For this review, use the dimensioned drawing (mm, ordinates from the lowest corner) and the shaded views. A direction names the side the tool comes from. Coordinates: 2 decimals unless noted, no trailing zeros. Order: outer loops, then holes, each group sorted by start corner. A loop starts at its lowest first (then second) coordinate and runs counter-clockwise, first axis right, second up. Notation, with made-up numbers: M 70.5,-3 L 121.5,-3 A28 ccw 121.5,15 Z; hole C 54.25,72.5 d1. An arc over 180 degrees is marked long. Use CSV: the item, a comma, the result in double quotes.
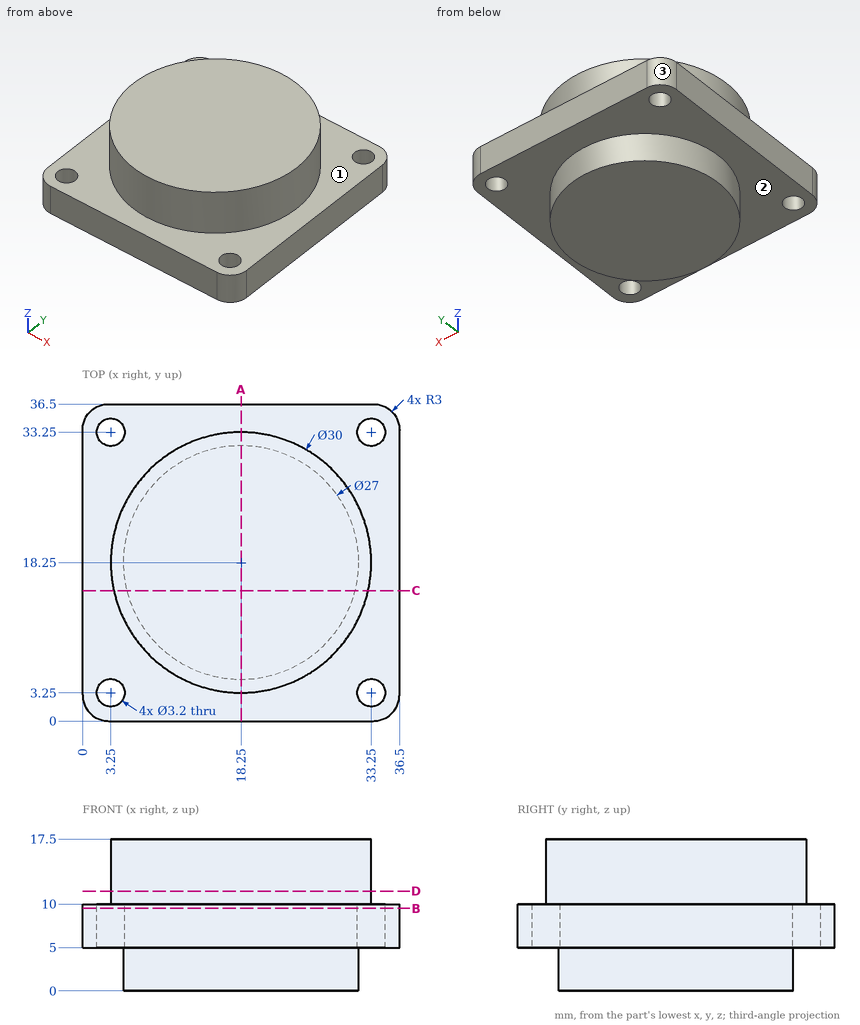
Item 1: Add section B-B on z = 9.5. State the section outline as (x, y) points.
Solutions:
outline,"M 0,3 A3 ccw 3,0 L 33.5,0 A3 ccw 36.5,3 L 36.5,33.5 A3 ccw 33.5,36.5 L 3,36.5 A3 ccw 0,33.5 Z; hole C 3.25,3.25 d3.2; hole C 3.25,33.25 d3.2; hole C 33.25,3.25 d3.2; hole C 33.25,33.25 d3.2"
Item 2: Add section C-C on y = 15. State the section outline as (x, z) points, and give its area (3 significant figures).
Solutions:
outline,"M 0,5 L 5.15,5 L 5.15,0 L 31.35,0 L 31.35,5 L 36.5,5 L 36.5,10 L 32.89,10 L 32.89,17.5 L 3.61,17.5 L 3.61,10 L 0,10 Z"
area,"533 mm^2"
Item 3: For the marked faces 1, 2 and 3, list the 3-axis set-ups (+Z, -Z, +X, -X, +Y, -Y) from which the entire face can be reached by the end or side of a thin tool; tool diameter is ignored.
Solutions:
face 1,"+Z"
face 2,"-Z"
face 3,"+Z, -Z, -X, +Y"
Item 4: To check wall thickness, follow line 1 along Y through (x, z) = (3.25, 8.3); line 2 along Z through (x, y) = (25, 33); line 3 along X through (y, z) = (2, 8). State the ranges of each line that lie inside material, in increasing order. Write a range as [from, to].
Solutions:
line 1,"[0, 1.65], [4.85, 31.65], [34.85, 36.5]"
line 2,"[5, 10]"
line 3,"[0.17, 2.25], [4.25, 32.25], [34.25, 36.33]"
Item 5: Clearance check with flat-ended pins moving along their axes: pin 1 Ø3.5 at (x, y) = (3.25, 3.25) entering from -Z; pin 2 Ø2 at (x, z) = (4.5, 14) entering from +Y; pin 3 Ø3 at (y, z) = (11, 12) entering from -X. State where each tip first meets the part, or that it passes through.
Solutions:
pin 1,"z = 5"
pin 2,"y = 26.15"
pin 3,"x = 4.4"
Item 6: Add section A-A on x = 18.25. State the section outline as (y, z) points, and give its area (4 significant figures).
Solutions:
outline,"M 0,5 L 4.75,5 L 4.75,0 L 31.75,0 L 31.75,5 L 36.5,5 L 36.5,10 L 33.25,10 L 33.25,17.5 L 3.25,17.5 L 3.25,10 L 0,10 Z"
area,"542.5 mm^2"
Item 7: Add section D-D on z = 11.5. State the section outline as (x, y) points, and give its area (3 significant figures).
Solutions:
outline,"C 18.25,18.25 d30"
area,"707 mm^2"
